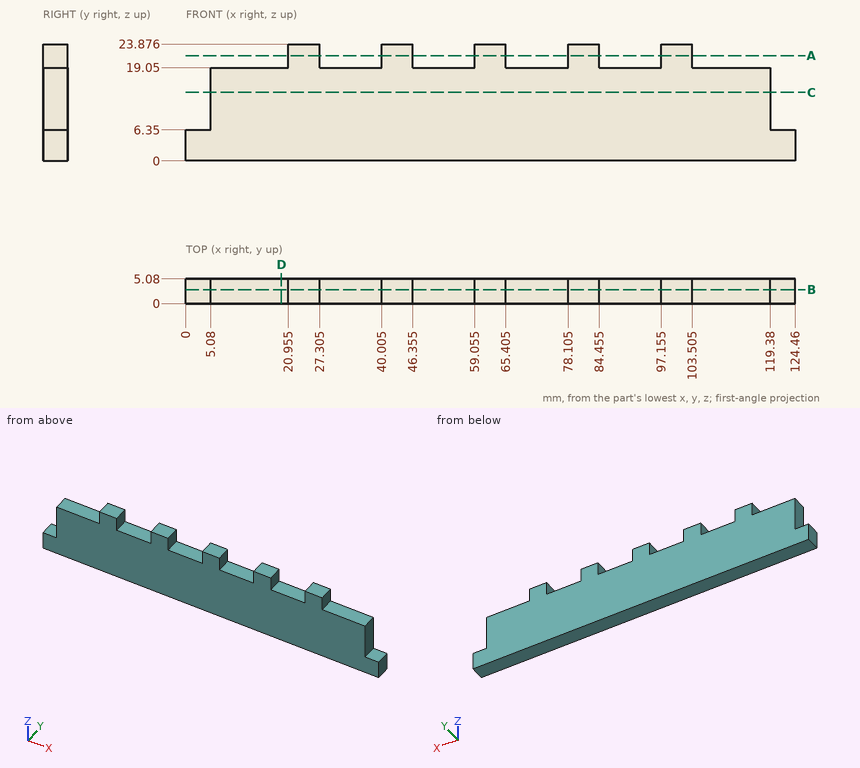
Verification items for this drawing (mm, ordinates from the low corner). Give positions to 0.01 mm unless a question says otherwise; leave off trailing zeros. Loops run counter-clockwise (first coordinate to the right, second up) from the corner with the lowest first, then second, coordinate; pieces in that order, holes last.
(1) Thickness scan on L1, parallel to X at y = 3.7, z = 10; L2, parallel to Z at x = 118.5, y = 4.9. Record the ranges inside material, lowest first.
From the geometry:
L1: x = 5.08 to 119.38
L2: z = 0 to 19.05
(2) Section check C-C on z = 14. Record the cut outline in (x, y), then the cut area to 3 significant figures.
From the geometry:
outline: (5.08, 0) - (119.38, 0) - (119.38, 5.08) - (5.08, 5.08) - close
area: 581 mm2
(3) Section check A-A on z = 21.5. Record the cut outline in (x, y) (3 decimals), then the cut area to 3 significant figures.
From the geometry:
outline: (20.955, 0) - (27.305, 0) - (27.305, 5.08) - (20.955, 5.08) - close; (40.005, 0) - (46.355, 0) - (46.355, 5.08) - (40.005, 5.08) - close; (59.055, 0) - (65.405, 0) - (65.405, 5.08) - (59.055, 5.08) - close; (78.105, 0) - (84.455, 0) - (84.455, 5.08) - (78.105, 5.08) - close; (97.155, 0) - (103.505, 0) - (103.505, 5.08) - (97.155, 5.08) - close
area: 161 mm2
(4) Section check D-D on x = 19.5. Record the cut outline in (y, z), then the cut area to 3 significant figures.
From the geometry:
outline: (0, 0) - (5.08, 0) - (5.08, 19.05) - (0, 19.05) - close
area: 96.8 mm2
(5) Depth check by flat-ended pin: pin 1 Ø2 at (y, z) = (1, 10.5) entering from -X; pin 2 Ø2.5 at (y, z) = (2, 22) entering from -X (3 decimals); pin 3 Ø2.5 at (y, z) = (2, 22.5) entering from +X (3 decimals). Enter the tip coordinate at first touch or a pass-through.
From the geometry:
pin 1: stops at x = 5.08
pin 2: stops at x = 20.955
pin 3: stops at x = 103.505
(6) Section check B-B on y = 2.9. Record the cut outline in (x, z) (3 decimals).
From the geometry:
outline: (0, 0) - (124.46, 0) - (124.46, 6.35) - (119.38, 6.35) - (119.38, 19.05) - (103.505, 19.05) - (103.505, 23.876) - (97.155, 23.876) - (97.155, 19.05) - (84.455, 19.05) - (84.455, 23.876) - (78.105, 23.876) - (78.105, 19.05) - (65.405, 19.05) - (65.405, 23.876) - (59.055, 23.876) - (59.055, 19.05) - (46.355, 19.05) - (46.355, 23.876) - (40.005, 23.876) - (40.005, 19.05) - (27.305, 19.05) - (27.305, 23.876) - (20.955, 23.876) - (20.955, 19.05) - (5.08, 19.05) - (5.08, 6.35) - (0, 6.35) - close
